Geometry: final body of the model. Coordinates: model frame, mm. A direction names the side the tool comes from. Give positions to 0.01 mm unless a question says otherwise; leave off trailing zeros. Loops run counter-clockwise (first coordinate to the right, second up) from the corner with the lowest first, then second, coordinate; pieces in that order, holes last. Notation, with made-up numbers: (33, 31.5) - (78, 31.5) arc R32 ccw to (78, 65.5) - close; hole circle Ø5 at (31.5, 52.25). An arc over 180 degrees is marked (long way). Answer in a Markdown table with one row per item.
from build123d import *

# Parameters (mm, degrees)
BLANKSKE_W              = 140
BLANKSKE_H              = 13
BLANK_DEPTH             = 5
TOOTHCUTSIM_DEPTH       = 141.691151108
TEETHCUTS_COUNT         = 45
TEETHCUTS_PITCH         = 3.14159265
SKETCH1_R               = 2.75
CUT_EXTRUDE2_DEPTH      = 141.691151108
CUT_EXTRUDE2_DEPTH_BACK = 10
SKETCH15_W              = 6
SKETCH15_H              = 5
BOSS_EXTRUDE4_DEPTH     = 5
SKETCH16_W              = 28
SKETCH16_H              = 28
BOSS_EXTRUDE5_DEPTH     = 7
CUT_EXTRUDE6_DEPTH      = 10
CHAMFER4_SIZE           = 3
CHAMFER5_SIZE           = 10
SKETCH18_R              = 1.35
CUT_EXTRUDE7_DEPTH      = 10


with BuildPart() as part:
    # BlankSke → Blank (new body)
    with BuildSketch(Plane.XY):
        with Locations((70, 6.5)):
            Rectangle(BLANKSKE_W, BLANKSKE_H)
    extrude(amount=-BLANK_DEPTH)

    # TooCutSkeSim → ToothCutSim (cut, through all)
    with BuildSketch(Plane.XY):
        Polygon((0.44443537, 10.75), (-0.44443537, 10.75), (-1.272613241, 13.0254), (1.272613241, 13.0254), align=None)
    toothcutsim = extrude(amount=-TOOTHCUTSIM_DEPTH, mode=Mode.SUBTRACT)

    # TeethCuts: ToothCutSim ×45
    with Locations(*[(i * TEETHCUTS_PITCH, 0, 0) for i in range(1, TEETHCUTS_COUNT)]):
        add(toothcutsim, mode=Mode.SUBTRACT)

    # Sketch1 → Cut-Extrude2 (cut, two sides)
    with BuildSketch(Plane(origin=(0, 0, 0), x_dir=(0, 0, -1), z_dir=(1, 0, 0))) as cut_extrude2_sk:
        with Locations((6, 4.5)):
            Circle(SKETCH1_R)
        with Locations((-1, 4.5)):
            Circle(SKETCH1_R)
    extrude(amount=CUT_EXTRUDE2_DEPTH, mode=Mode.SUBTRACT)
    extrude(cut_extrude2_sk.sketch, amount=-CUT_EXTRUDE2_DEPTH_BACK, mode=Mode.SUBTRACT)

    # Sketch15 → Boss-Extrude4 (add)
    with BuildSketch(Plane.XZ):
        with Locations((3, -2.5)):
            Rectangle(SKETCH15_W, SKETCH15_H)
    extrude(amount=BOSS_EXTRUDE4_DEPTH)

    # Sketch16 → Boss-Extrude5 (add)
    with BuildSketch(Plane.ZY):
        with Locations((-2.5, -19)):
            Rectangle(SKETCH16_W, SKETCH16_H)
    extrude(amount=-BOSS_EXTRUDE5_DEPTH)

    # Sketch17 → Cut-Extrude6 (cut)
    with BuildSketch(Plane.ZY):
        Polygon((-13.813708499, -19), (-2.5, -7.686291501), (8.813708499, -19), (-2.5, -30.313708499), align=None)
    extrude(amount=-CUT_EXTRUDE6_DEPTH, mode=Mode.SUBTRACT)

    # Chamfer4
    chamfer4_edges = [part.edges().sort_by_distance(p)[0] for p in [
        (3.5, -30.313708499, -2.5),
    ]]
    chamfer(chamfer4_edges, length=CHAMFER4_SIZE)

    # Chamfer5
    chamfer5_edges = [part.edges().sort_by_distance(p)[0] for p in [
        (3.5, -5, 11.5),
        (3.5, -33, 11.5),
        (3.5, -33, -16.5),
        (3.5, -5, -16.5),
    ]]
    chamfer(chamfer5_edges, length=CHAMFER5_SIZE)

    # Sketch18 → Cut-Extrude7 (cut)
    with BuildSketch(Plane.XZ.offset(33)):
        with Locations(Location((3.5, -2.5, 0), (0, 0, 270))):
            Circle(SKETCH18_R)
    extrude(amount=-CUT_EXTRUDE7_DEPTH, mode=Mode.SUBTRACT)


solid = part.part
Q1. First-contact query: pin 1 (3 mm diameter, centred on y = -27.5, z = 0.5, fed in from +X); pin 2 (7.5 mm diameter, centred on x = 73.5, y = -2, fed in from +Z); pin 3 (5 mm diameter, centred on x = 121.5, y = -2, fed in from -Z). Flat tips, straight axial feed; report the tip coordinate or a pass-through.
Check values:
| item | result |
|---|---|
| pin 1 | x = 7 |
| pin 2 | z = 0 |
| pin 3 | z = -5 |
Q2. Reachability of faces 1 (the flat face through (0, -12.6, -7.8)), 2 (the flat face through (124.8, 11.9, -2.5)), 3 (the flat face through (3.5, -5, -5.2)) from +Z, -Z, +X, -X, +Y, -Y: full face, straight path, thin tool, end or side. Return the list, or none.
Check values:
| item | result |
|---|---|
| face 1 | +Z, -Z, -X, +Y, -Y |
| face 2 | +Z, -Z, +Y |
| face 3 | +X |
Q3. Cut plane A-A (y = -24.5). Output: boundary loops of the cut face in (x, z).
Check values:
| item | result |
|---|---|
| outline | (0, -15) - (7, -15) - (7, -8.31) - (0, -8.31) - close; (0, 3.31) - (7, 3.31) - (7, 10) - (0, 10) - close |
Q4. Material intervals for line 1 along X through (y, z) = (-30.35, -2.5); line 2 along Y through (x, z) = (33, -4); line 3 along Z through (x, y) = (3, -29), sorted ascending.
Check values:
| item | result |
|---|---|
| line 1 | 0 to 2.15, 4.85 to 7 |
| line 2 | 0 to 2.61, 6.39 to 13 |
| line 3 | -10.5 to -3.75, -1.25 to 5.5 |
